The model under review builds one solid part; all positions refer to its coordinate system, in mm. A direction names the side the tool comes from. Round coordinates to 2 decimals unless told otherwise and drop trailing zeros. Loops run counter-clockwise (first coordinate to the right, second up) from the corner with the lowest first, then second, coordinate; pieces in that order, holes last. Notation, with made-up numbers: M 5.25,-24 L 15.25,-24 A9 ccw 15.25,-20 Z; hole C -35.75,27.25 d10. An arc over 180 degrees is marked long. Answer in a Markdown table with one row per item. Add a question column.
from build123d import *

# Parameters (mm, degrees)
F0_W      = 40
F0_H      = 35.9344822692
F1_DEPTH  = 20
F2_W      = 28
F2_H      = 14
F3_DEPTH  = 5
F4_W      = 14
F4_H      = 1.12
F5_DEPTH  = 3
F6_W      = 3
F6_H      = 1
F7_DEPTH  = 0.5
F8_W      = 12
F8_H      = 14
F9_DEPTH  = 2.5
F10_DEPTH = 25
F11_W     = 9.0484669507
F11_H     = 1.2658234112
F11_H_2   = 5.2294719476
F12_DEPTH = 2.5
F13_W     = 40
F13_H     = 1.2
F14_DEPTH = 0.5
F15_W     = 40
F15_H     = 1.2
F16_DEPTH = 0.5
F17_DEPTH = 2.5


with BuildPart() as f1:
    # F0 (on Top) → F1 (new body)
    with BuildSketch(Plane.XY):
        Rectangle(F0_W, F0_H)
    extrude(amount=F1_DEPTH)

    # F2 (on face) → F3 (cut)
    with BuildSketch(Plane.XY.offset(20)):
        with Locations((6, 0)):
            Rectangle(F2_W, F2_H)
    extrude(amount=-F3_DEPTH, mode=Mode.SUBTRACT)

    # F4 (on face) → F5 (cut)
    with BuildSketch(Plane.YZ.offset(-8)):
        with Locations((0, 15.56)):
            Rectangle(F4_W, F4_H)
    extrude(amount=-F5_DEPTH, mode=Mode.SUBTRACT)

    # F6 (on face) → F7 (cut)
    with BuildSketch(Plane(origin=(0, 0, 16.12), x_dir=(1, 0, 0), z_dir=(0, 0, -1))):
        with Locations((-9.5, -3.5)):
            Rectangle(F6_W, F6_H)
        with Locations((-9.5, -2.25)):
            Rectangle(F6_W, F6_H)
        with Locations((-9.5, -1)):
            Rectangle(F6_W, F6_H)
        with Locations((-9.5, 0.25)):
            Rectangle(F6_W, F6_H)
    extrude(amount=-F7_DEPTH, mode=Mode.SUBTRACT)

    # F8 (on face) → F9 (cut)
    with BuildSketch(Plane.XY.offset(20)):
        with Locations((-14, 0)):
            Rectangle(F8_W, F8_H)
    extrude(amount=-F9_DEPTH, mode=Mode.SUBTRACT)

    # F10 (cut): a face of the model
    f10_faces = [f1.faces().sort_by_distance(p)[0] for p in [
        (-11, 0.1838235294, 15.6516289593),
    ]]
    extrude(f10_faces, amount=-F10_DEPTH, mode=Mode.SUBTRACT)

    # F11 (on face) → F12 (cut, through all)
    with BuildSketch(Plane.XY.offset(17.5)):
        with Locations((-12.5242334753, 6.3670882944)):
            Rectangle(F11_W, F11_H)
        with Locations((-12.5242334753, -4.3852640262)):
            Rectangle(F11_W, F11_H_2)
    extrude(amount=-F12_DEPTH, mode=Mode.SUBTRACT)

    # F13 (on face) → F14 (cut)
    with BuildSketch(Plane(origin=(0, -7, 0), x_dir=(-1, 0, 0), z_dir=(0, 1, 0))):
        with Locations((0, 15.6)):
            Rectangle(F13_W, F13_H)
    extrude(amount=-F14_DEPTH, mode=Mode.SUBTRACT)

    # F15 (on face) → F16 (cut)
    with BuildSketch(Plane.XZ.offset(-7)):
        with Locations((0, 15.6)):
            Rectangle(F15_W, F15_H)
    extrude(amount=-F16_DEPTH, mode=Mode.SUBTRACT)

    # F17 (cut, through all): a face of the model
    f17_faces = [f1.faces().sort_by_distance(p)[0] for p in [
        (-14.7940711772, 1.2320876945, 17.5),
    ]]
    extrude(f17_faces, amount=-F17_DEPTH, mode=Mode.SUBTRACT)


solid = f1.part
1. To check wall thickness, follow probe 1 along Y at (x, z) = (1, 15.25); probe 2 along Y at (x, z) = (4, 17.25); probe 3 along Z at (x, y) = (5, 4). State the ranges of each line that lie inside material, in increasing order.
2. Take a section at C-C, the plane y = 0. State the section outline as (x, z) points.
3. Machinability: for faces 5 (the flat face through (20, 0, 10)), 6 (the flat face through (0, 7.5, 16)), 7 (the flat face through (0, -7, 18)), which of the approach directions +Z, -Z, +X, -X, +Y, -Y give a long, thin tool a straight path to every point of the face, cutting with its end or side? Answer none if there is none.
4. Take a section at A-A, the plane z = 18.25. State the section outline as (x, y) points.
5. Mouldability with a two-part tool opening along Y and no side actions: class faces 1 (the flat face through (0, -7.5, 16)), 2 (the flat face through (0, 17.967, 10)), 3 (the flat face through (0, 13, 20)), 4 (the flat face through (0, -17.967, 10)) as released by +Y, released by -Y, zero draft, split by the parting line, or undercut.
6. Take a section at B-B, the plane x = -10.5. State the section outline as (y, z) points, and give its area (3 significant figures).
7. For pin 1 Ø4.5 at (x, y) = (3, 3) entering from +Z; pin 2 Ø0.6 at (x, y) = (0.5, -7.5) entering from -Z, all flat-tipped, find the tip position at first contact; note any pin that passes through.
Check sheet entries:
| question | item | result |
|---|---|---|
| 1 | probe 1 | y = -17.97 to -7.5, 7.5 to 17.97 |
| 1 | probe 2 | y = -17.97 to -7, 7 to 17.97 |
| 1 | probe 3 | z = 0 to 15 |
| 2 | outline | M -20,0 L 20,0 L 20,15 L -20,15 Z |
| 3 | face 5 | +Z, -Z, +X, +Y, -Y |
| 3 | face 6 | +X, -X |
| 3 | face 7 | +Z, +X, -X |
| 4 | outline | M -20,-17.97 L 20,-17.97 L 20,-7 L -20,-7 Z; M -20,7 L 20,7 L 20,17.97 L -20,17.97 Z |
| 5 | face 1 | undercut |
| 5 | face 2 | released by +Y |
| 5 | face 3 | zero draft |
| 5 | face 4 | released by -Y |
| 6 | outline | M -17.97,0 L 17.97,0 L 17.97,20 L 7,20 L 7,16.2 L 7.5,16.2 L 7.5,15 L -7.5,15 L -7.5,16.2 L -7,16.2 L -7,20 L -17.97,20 Z |
| 6 | area | 647 mm^2 |
| 7 | pin 1 | stops at z = 15 |
| 7 | pin 2 | stops at z = 0 |
